Design review of the part built by this model. Coordinates are the model's own, in mm. Round coordinates to 2 decimals unless told otherwise and drop trailing zeros. Order: outer loops, then holes, each group sorted by start corner. A loop starts at its lowest first (then second) coordinate and runs counter-clockwise, first axis right, second up. Notation, with made-up numbers: (36.5, 21.25) - (78.5, 21.25) arc R25 cw to (78.5, 49.25) - close; hole circle Ø10 at (13.5, -19.5). An arc over 180 degrees is marked (long way). Write item = value, one per line.
from build123d import *

# Parameters (mm, degrees)
SKETCH_1_R      = 28
EXTRUDE_1_DEPTH = 2
SKETCH_2_W      = 15
SKETCH_2_H      = 15
EXTRUDE_2_DEPTH = 1.5
SKETCH_4_W      = 10
SKETCH_4_H      = 20
EXTRUDE_3_DEPTH = 1.5
SKETCH_5_W      = 15
SKETCH_5_H      = 15
EXTRUDE_4_DEPTH = 1.5


with BuildPart() as part:
    # 草图1 → 凸台-拉伸1 (new body)
    with BuildSketch(Plane.XY):
        Circle(SKETCH_1_R)
    extrude(amount=EXTRUDE_1_DEPTH)

    # 草图2 → 凸台-拉伸2 (add)
    with BuildSketch(Plane.XY.offset(2)):
        Rectangle(SKETCH_2_W, SKETCH_2_H)
    extrude(amount=EXTRUDE_2_DEPTH)

    # 草图4 → 凸台-拉伸3 (add)
    with BuildSketch(Plane(origin=(0, 0, 0), x_dir=(-1, 0, 0), z_dir=(0, 0, -1))):
        with Locations((19, 0)):
            Rectangle(SKETCH_4_W, SKETCH_4_H)
    extrude(amount=EXTRUDE_3_DEPTH)

    # 草图5 → 凸台-拉伸4 (add)
    with BuildSketch(Plane(origin=(0, 0, 0), x_dir=(-1, 0, 0), z_dir=(0, 0, -1))):
        Rectangle(SKETCH_5_W, SKETCH_5_H)
    extrude(amount=EXTRUDE_4_DEPTH)


solid = part.part
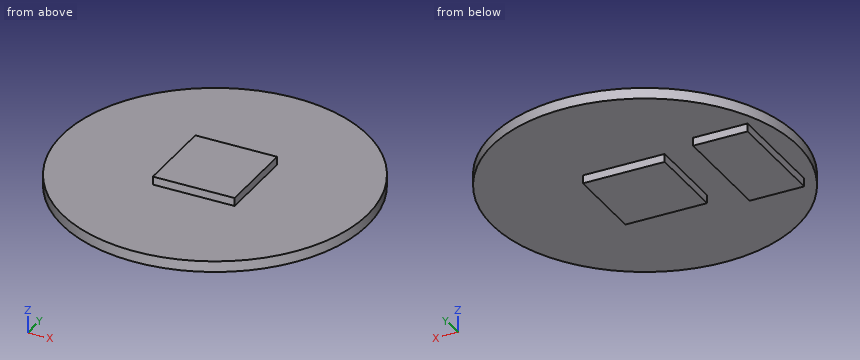
1) To check wall thickness, follow L1, parallel to X at y = -2.5, z = -1.3; L2, parallel to Z at x = 21, y = -9; L3, parallel to Y at x = -6.5, z = -0.8. State the ranges of each line that lie inside material, in increasing order. Write a range as from..to.
Findings:
L1 = -24..-14, -7.5..7.5
L2 = 0..2
L3 = -7.5..7.5
2) We need section B-B on y = 0. Write out the cut boundary in (x, z).
Findings:
outline = (-28, 0) - (-24, 0) - (-24, -1.5) - (-14, -1.5) - (-14, 0) - (-7.5, 0) - (-7.5, -1.5) - (7.5, -1.5) - (7.5, 0) - (28, 0) - (28, 2) - (7.5, 2) - (7.5, 3.5) - (-7.5, 3.5) - (-7.5, 2) - (-28, 2) - close
3) We need section A-A on x = 0. Write out the cut boundary in (y, z), and give its area (3 significant figures).
Findings:
outline = (-28, 0) - (-7.5, 0) - (-7.5, -1.5) - (7.5, -1.5) - (7.5, 0) - (28, 0) - (28, 2) - (7.5, 2) - (7.5, 3.5) - (-7.5, 3.5) - (-7.5, 2) - (-28, 2) - close
area = 157 mm^2
4) Clearance check with flat-ended pins moving along their axes: pin 1 Ø0.8 at (x, z) = (-3, 2.5) entering from -Y; pin 2 Ø1 at (x, y) = (-2, -9) entering from -Z; pin 3 Ø1.6 at (x, z) = (-1, 3) entering from +Y. State where each tip first meets the part, or that it passes through.
Findings:
pin_1 = -7.5
pin_2 = 0
pin_3 = 7.5
5) We need section D-D on y = 6. Write out the cut boundary in (x, z), and give its area (3 significant figures).
Findings:
outline = (-27.35, 0) - (-24, 0) - (-24, -1.5) - (-14, -1.5) - (-14, 0) - (-7.5, 0) - (-7.5, -1.5) - (7.5, -1.5) - (7.5, 0) - (27.35, 0) - (27.35, 2) - (7.5, 2) - (7.5, 3.5) - (-7.5, 3.5) - (-7.5, 2) - (-27.35, 2) - close
area = 169 mm^2
6) We need section C-C on z = 2.75. Write out the cut boundary in (x, y).
Findings:
outline = (-7.5, -7.5) - (7.5, -7.5) - (7.5, 7.5) - (-7.5, 7.5) - close
